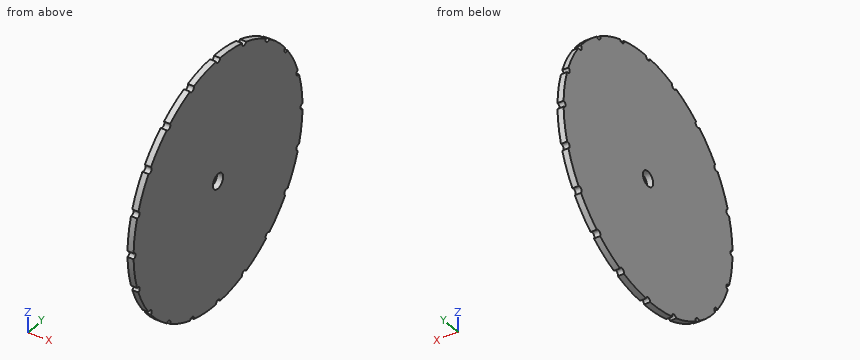
from build123d import *

# Parameters (mm, degrees)
F0_R            = 82.5
F0_R_2          = 5
F1_DEPTH        = 2
F1_DEPTH_BACK   = 2
F2_R            = 2
F3_DEPTH        = 4.001
F3_COPIES_COUNT = 20


# Not quite as in the source:
# - a pattern or mirror of a feature is missing from the dataset's text; its kind, count and spacing are read off the source's solid


with BuildPart() as f1:
    # F0 (on Right) → F1 (new body, two sides)
    with BuildSketch(Plane.YZ) as f1_sk:
        Circle(F0_R)
        Circle(F0_R_2, mode=Mode.SUBTRACT)
    extrude(amount=F1_DEPTH)
    extrude(f1_sk.sketch, amount=-F1_DEPTH_BACK)

    # F2 (on face) → F3 (cut, through all)
    with BuildSketch(Plane.YZ.offset(2)):
        with Locations((0, 82.5)):
            Circle(F2_R)
    f3 = extrude(amount=-F3_DEPTH, mode=Mode.SUBTRACT)

    # F3_copies: F3 ×20 about axis
    f3_copies_axis = Axis((0, 0, 0), (1, 0, 0))
    for i in range(1, F3_COPIES_COUNT):
        add(f3.rotate(f3_copies_axis, i * 360 / F3_COPIES_COUNT), mode=Mode.SUBTRACT)


solid = f1.part
For this review, take the finished solid that the model builds, in its own axes (mm). Give positions to 0.01 mm unless a question says otherwise; leave off trailing zeros. Write each loop counter-clockwise with the first axis right and the second up, starting at its lowest first coordinate (ties: lowest second). Pieces come first, ordered by that corner, then holes. Notation, with made-up numbers: (-3.75, -17) -> (19.25, -17) arc R26 cw to (19.25, 20) -> close; hole circle Ø5 at (-29, 22.5). An arc over 180 degrees is marked (long way). Use CSV: the item, a comma, the result in double quotes.
Q1. To check wall thickness, follow probe 1 along Z at (x, y) = (0.9, 0); probe 2 along Z at (x, y) = (-1.6, -2.5); probe 3 along Y at (x, z) = (-0.05, 65). State the ranges of each line that lie inside material, in increasing order. Write a range as [from, to].
Conclusion:
probe 1,"[-80.5, -5], [5, 80.5]"
probe 2,"[-82.46, -4.33], [4.33, 82.46]"
probe 3,"[-50.81, -49.47], [-47.51, 47.51], [49.47, 50.81]"
Q2. For P1, Ø1, axis at x = 0.5, y = -58.5, coming from the -Z side; P2, Ø1.5, axis at x = 0, y = -20, coming from the -Z side; P3, Ø11.5, axis at y = 0, z = 0, coming from the +X side; P4, Ø1, axis at x = -0.5, z = 26.5, coming from the +Y side, all flat-tipped, find the tip position at first contact; note any pin that passes through.
Conclusion:
P1,"z = -58.67"
P2,"z = -80.22"
P3,"x = 2"
P4,"y = 77.15"
Q3. Take a section at C-C, the plane y = -17. Write out the cut boundary in (x, z).
Conclusion:
outline,"(-2, -80.73) -> (2, -80.73) -> (2, 80.73) -> (-2, 80.73) -> close"
Q4. Take a section at A-A, the plane z = 0. Write out the cut boundary in (x, y).
Conclusion:
outline,"(-2, -80.5) -> (2, -80.5) -> (2, -5) -> (-2, -5) -> close; (-2, 5) -> (2, 5) -> (2, 80.5) -> (-2, 80.5) -> close"
Q5. Take a section at D-D, the plane z = 30.5. Write out the cut boundary in (x, y).
Conclusion:
outline,"(-2, -76.66) -> (2, -76.66) -> (2, 76.66) -> (-2, 76.66) -> close"
